from build123d import *

# Parameters (mm, degrees)
F0_R      = 2.286
F1_DEPTH  = 2.286
F1_FACE_R = 2.286
F2_DEPTH  = 2.286
F3_R      = 6.731
F4_DEPTH  = 1.524
F5_R      = 6.731
F6_DEPTH  = 1.524


with BuildPart() as f1:
    # F0 (on Front) → F1 (new body)
    with BuildSketch(Plane.XZ):
        Circle(F0_R)
    extrude(amount=F1_DEPTH)

    # F1_face (on face) → F2 (join)
    with BuildSketch(Plane(origin=(0, 0, 0), x_dir=(1, 0, 0), z_dir=(0, 1, 0))):
        Circle(F1_FACE_R)
    extrude(amount=F2_DEPTH)

    # F3 (on face) → F4 (join)
    with BuildSketch(Plane(origin=(0, 2.286, 0), x_dir=(-1, 0, 0), z_dir=(0, 1, 0))):
        Circle(F3_R)
    extrude(amount=F4_DEPTH)

    # F5 (on face) → F6 (join)
    with BuildSketch(Plane.XZ.offset(2.286)):
        Circle(F5_R)
    extrude(amount=F6_DEPTH)


solid = f1.part
Input: part model. Units: mm. Frame: model coordinates. A direction names the side the tool comes from. Coordinates: 2 decimals unless noted, no trailing zeros. Order: outer loops, then holes, each group sorted by start corner. A loop starts at its lowest first (then second) coordinate and runs counter-clockwise, first axis right, second up. Notation, with made-up numbers: M -18.5,15 L -12.5,15 A17 ccw -12.5,33 Z; hole C 85,73.25 d6. An arc over 180 degrees is marked long. Write item = value, one per line. Start each with the question number.
(1) First-contact query: P1, Ø1.5, axis at x = -5.5, y = 2, coming from the -Z side; P2, Ø2, axis at y = -2, z = -2.5, coming from the -X side. Flat tips, straight axial feed; report the tip coordinate or a pass-through.
(2) Section A-A on z = 0. Output: boundary loops of the cut face in (x, y), and give its area (3 significant figures).
(3) Pull-direction query (Y, two-part tool) for faces 3 (the cylindrical face through (-0.5, -0.03, 2.23)), 4 (the cylindrical face through (5.34, 3.04, -4.1)), 5 (the flat face through (0, -3.81, 0)); classes: released by +Y, released by -Y, zero draft, split by the parting line, or undercut.
(4) Section C-C on z = 4. Output: boundary loops of the cut face in (x, y).
(5) Section D-D on x = 0. Output: boundary loops of the cut face in (y, z), and give its area (3 significant figures).
(6) Line query: line 1 along Y through (x, z) = (0.75, -3.5); line 2 along X through (y, z) = (0.5, -0.5); line 3 along Z through (x, y) = (-2, 2). Output: solid intervals per line, ascending. Write a range as [from, to].
(7) Reachability of faces 1 (the cylindrical face through (-5.34, -3.04, -4.1)), 2 (the flat face through (-3, 2.286, 0)) from +Z, -Z, +X, -X, +Y, -Y: full face, straight path, thin tool, end or side. Return the list, or none.
(8) Section B-B on x = -5.25. Output: boundary loops of the cut face in (y, z).
Result set:
q1.P1 = -4.71
q1.P2 = -6.55
q2.outline = M -6.73,-3.81 L 6.73,-3.81 L 6.73,-2.29 L 2.29,-2.29 L 2.29,2.29 L 6.73,2.29 L 6.73,3.81 L -6.73,3.81 L -6.73,2.29 L -2.29,2.29 L -2.29,-2.29 L -6.73,-2.29 Z
q2.area = 61.9 mm²
q3.face_3 = undercut
q3.face_4 = zero draft
q3.face_5 = released by -Y
q4.outline = M -5.41,-3.81 L 5.41,-3.81 L 5.41,-2.29 L -5.41,-2.29 Z; M -5.41,2.29 L 5.41,2.29 L 5.41,3.81 L -5.41,3.81 Z
q5.outline = M -3.81,-6.73 L -2.29,-6.73 L -2.29,-2.29 L 2.29,-2.29 L 2.29,-6.73 L 3.81,-6.73 L 3.81,6.73 L 2.29,6.73 L 2.29,2.29 L -2.29,2.29 L -2.29,6.73 L -3.81,6.73 Z
q5.area = 61.9 mm²
q6.line_1 = [-3.81, -2.29], [2.29, 3.81]
q6.line_2 = [-2.23, 2.23]
q6.line_3 = [-1.11, 1.11]
q7.face_1 = +Y, -Y
q7.face_2 = none
q8.outline = M -3.81,-4.21 L -2.29,-4.21 L -2.29,4.21 L -3.81,4.21 Z; M 2.29,-4.21 L 3.81,-4.21 L 3.81,4.21 L 2.29,4.21 Z
